from build123d import *

# Parameters (mm, degrees)
SKETCH1_W               = 147.6
SKETCH1_H               = 78.1
BOSS_EXTRUDE1_DEPTH     = 14.5
SKETCH2_W               = 112
SKETCH2_H               = 78.1
BOSS_EXTRUDE2_DEPTH     = 93.5
CUT_EXTRUDE1_REACH      = 200.87
CUT_EXTRUDE2_DEPTH      = 8.4
CUT_EXTRUDE2_DEPTH_BACK = 8.4
SKETCH4_R               = 6.5
CUT_EXTRUDE3_REACH      = 185.305
SKETCH5_R               = 4
SKETCH7_R               = 4
CUT_EXTRUDE4_DEPTH      = 199.870234166


with BuildPart() as part:
    # Sketch1 → Boss-Extrude1 (new body)
    with BuildSketch(Plane.XY):
        with Locations((73.8, 39.05)):
            Rectangle(SKETCH1_W, SKETCH1_H)
    extrude(amount=BOSS_EXTRUDE1_DEPTH)

    # Sketch2 → Boss-Extrude2 (add)
    with BuildSketch(Plane.XY.offset(14.5)):
        with Locations((73.8, 39.05)):
            Rectangle(SKETCH2_W, SKETCH2_H)
    extrude(amount=BOSS_EXTRUDE2_DEPTH)

    # Sketch3 → Cut-Extrude1 (cut, up to next)
    with BuildSketch(Plane(origin=(0, 78.1, 0), x_dir=(1, 0, 0), z_dir=(0, 1, 0)), mode=Mode.PRIVATE) as cut_extrude1_sk1:
        with BuildLine():
            Line((29.8, -84), (17.8, -84))
            Line((17.8, -84), (17.8, -108))
            Line((17.8, -108), (73.8, -108))
            ThreePointArc((73.8, -108), (48.740071828, -101.609868316), (29.8, -84))
        make_face()
    cut_extrude1_tool1 = extrude(cut_extrude1_sk1.sketch, amount=-CUT_EXTRUDE1_REACH, mode=Mode.PRIVATE) & part.part
    # Sketch3 → Cut-Extrude1 (cut, up to next)
    with BuildSketch(Plane(origin=(0, 78.1, 0), x_dir=(1, 0, 0), z_dir=(0, 1, 0)), mode=Mode.PRIVATE) as cut_extrude1_sk2:
        with BuildLine():
            Line((17.8, -53.866666667), (17.8, -57.466666667))
            Line((17.8, -57.466666667), (33.840520524, -57.466666667))
            ThreePointArc((33.840520524, -57.466666667), (113.8, -55.666666667), (33.840520524, -53.866666667))
            Line((33.840520524, -53.866666667), (17.8, -53.866666667))
        make_face()
    cut_extrude1_tool2 = extrude(cut_extrude1_sk2.sketch, amount=-CUT_EXTRUDE1_REACH, mode=Mode.PRIVATE) & part.part
    # Sketch3 → Cut-Extrude1 (cut, up to next)
    with BuildSketch(Plane(origin=(0, 78.1, 0), x_dir=(1, 0, 0), z_dir=(0, 1, 0)), mode=Mode.PRIVATE) as cut_extrude1_sk3:
        with BuildLine():
            ThreePointArc((117.8, -84), (98.859928172, -101.609868316), (73.8, -108))
            Line((73.8, -108), (129.8, -108))
            Line((129.8, -108), (129.8, -84))
            Line((129.8, -84), (117.8, -84))
        make_face()
    cut_extrude1_tool3 = extrude(cut_extrude1_sk3.sketch, amount=-CUT_EXTRUDE1_REACH, mode=Mode.PRIVATE) & part.part
    add(cut_extrude1_tool1.solids().sort_by_distance((32.341594, 78.1, 98.707997))[0], mode=Mode.SUBTRACT)
    add(cut_extrude1_tool2.solids().sort_by_distance((73.255815, 78.1, 55.666667))[0], mode=Mode.SUBTRACT)
    add(cut_extrude1_tool3.solids().sort_by_distance((115.258406, 78.1, 98.707997))[0], mode=Mode.SUBTRACT)

    # Sketch4 → Cut-Extrude2 (cut, two sides: drawn at the far end of the back side and taken through both)
    with BuildSketch(Plane.XY.offset(84).offset(-CUT_EXTRUDE2_DEPTH_BACK)):
        with Locations(Location((25.5, 61.05, 0), (0, 0, 311.417298986))):
            Circle(SKETCH4_R)
        with Locations(Location((25.5, 39.05, 0), (0, 0, 311.417298986))):
            Circle(SKETCH4_R)
        with Locations(Location((25.5, 17.05, 0), (0, 0, 180))):
            Circle(SKETCH4_R)
    extrude(amount=CUT_EXTRUDE2_DEPTH + CUT_EXTRUDE2_DEPTH_BACK, mode=Mode.SUBTRACT)

    # Sketch5 → Cut-Extrude3 (cut, up to next)
    with BuildSketch(Plane.XY.offset(75.6), mode=Mode.PRIVATE) as cut_extrude3_sk1:
        with Locations((25.5, 61.05)):
            Circle(SKETCH5_R)
    cut_extrude3_tool1 = extrude(cut_extrude3_sk1.sketch, amount=-CUT_EXTRUDE3_REACH, mode=Mode.PRIVATE) & part.part
    # Sketch5 → Cut-Extrude3 (cut, up to next)
    with BuildSketch(Plane.XY.offset(75.6), mode=Mode.PRIVATE) as cut_extrude3_sk2:
        with Locations((25.5, 39.05)):
            Circle(SKETCH5_R)
    cut_extrude3_tool2 = extrude(cut_extrude3_sk2.sketch, amount=-CUT_EXTRUDE3_REACH, mode=Mode.PRIVATE) & part.part
    # Sketch5 → Cut-Extrude3 (cut, up to next)
    with BuildSketch(Plane.XY.offset(75.6), mode=Mode.PRIVATE) as cut_extrude3_sk3:
        with Locations((25.5, 17.05)):
            Circle(SKETCH5_R)
    cut_extrude3_tool3 = extrude(cut_extrude3_sk3.sketch, amount=-CUT_EXTRUDE3_REACH, mode=Mode.PRIVATE) & part.part
    add(cut_extrude3_tool1.solids().sort_by_distance((25.5, 61.05, 75.6))[0], mode=Mode.SUBTRACT)
    add(cut_extrude3_tool2.solids().sort_by_distance((25.5, 39.05, 75.6))[0], mode=Mode.SUBTRACT)
    add(cut_extrude3_tool3.solids().sort_by_distance((25.5, 17.05, 75.6))[0], mode=Mode.SUBTRACT)

    # Sketch7 → Cut-Extrude4 (cut, through all)
    with BuildSketch(Plane(origin=(0, 0, 0), x_dir=(-1, 0, 0), z_dir=(0, 0, -1))):
        with Locations((-9, 63.1)):
            Circle(SKETCH7_R)
        with Locations((-9, 13.1)):
            Circle(SKETCH7_R)
        with Locations((-138.6, 13.1)):
            Circle(SKETCH7_R)
        with Locations((-138.6, 63.1)):
            Circle(SKETCH7_R)
    extrude(amount=-CUT_EXTRUDE4_DEPTH, mode=Mode.SUBTRACT)


solid = part.part
Source: CAD feature listing. Evaluate the final solid. Frame: model axes, mm. A direction names the side the tool comes from. Round coordinates to 2 decimals unless told otherwise and drop trailing zeros. Loops run counter-clockwise (first coordinate to the right, second up) from the corner with the lowest first, then second, coordinate; pieces in that order, holes last. Notation, with made-up numbers: (34.5, 0.5) - (56.5, 0.5) arc R18 cw to (56.5, 22.5) - close; hole circle Ø6 at (10.5, -14). An arc over 180 degrees is marked (long way). Write item = value, one per line. Start each with the question number.
Item 1: Reachability of faces 4 (the face through (31, 40, 57.467)), 5 (the face through (24.979, 43.016, 66.66)), 6 (the face through (17.8, 39, 34)) from +Z, -Z, +X, -X, +Y, -Y: full face, straight path, thin tool, end or side. Return the list, or none.
Item 2: Section query B-B on z = 31.5. Output: boundary loops of the cut face in (x, y).
Item 3: Section query A-A on x = 9. Output: boundary loops of the cut face in (y, z), plus the area to 3 significant figures.
Item 4: Section query D-D on y = 61.05. Count the separate pieces of the cut face and the enclosed holes in it, plus the area to 3 significant figures.
Item 5: Mould query, pull axis Z, two halves, no side actions, for faces 1 (the face through (26, 40, 53.867)), 2 (the face through (21, 17, 75.6)), 3 (the face through (0, 39, 7)). Classes: released by +Z, released by -Z, zero draft, split by the parting line, or undercut.
Item 6: Material intervals for line 1 (Y direction, x = 138.6, z = 3.75); line 2 (Y direction, x = 25, z = 78); line 3 (Z direction, x = 27.5, y = 72.5), sorted ascending.
Item 7: Section query C-C on y = 39.05. Output: boundary loops of the cut face in (x, z), plus the area to 3 significant figures.
Item 8: First-contact query: pin 1 Ø9 at (x, y) = (25.5, 17.05) entering from +Z; pin 2 Ø10 at (x, y) = (107, 51) entering from +Z; pin 3 Ø21 at (x, y) = (25.5, 17.05) entering from +Z. Flat tips, straight axial feed; report the tip coordinate or a pass-through.
Results list:
q1.face_4 = -X, +Y, -Y
q1.face_5 = +Z
q1.face_6 = +Z, -X, +Y, -Y
q2.outline = (17.8, 0) - (41.93, 0) - (41.93, 78.1) - (17.8, 78.1) - close; (105.67, 0) - (129.8, 0) - (129.8, 78.1) - (105.67, 78.1) - close
q3.outline = (0, 0) - (9.1, 0) - (9.1, 14.5) - (0, 14.5) - close; (17.1, 0) - (59.1, 0) - (59.1, 14.5) - (17.1, 14.5) - close; (67.1, 0) - (78.1, 0) - (78.1, 14.5) - (67.1, 14.5) - close
q3.area = 900 mm²
q4.separate_pieces = 4
q4.enclosed_holes = 0
q4.area = 5,870 mm²
q5.face_1 = undercut
q5.face_2 = released by +Z
q5.face_3 = zero draft
q6.line_1 = 0 to 9.1, 17.1 to 59.1, 67.1 to 78.1
q6.line_2 = 0 to 10.57, 23.53 to 32.57, 45.53 to 54.57, 67.53 to 78.1
q6.line_3 = 0 to 53.87, 57.47 to 84
q7.outline = (0, 0) - (147.6, 0) - (147.6, 14.5) - (129.8, 14.5) - (129.8, 84) - (117.8, 84) arc R52.33 ccw to (32, 87.16) - (32, 75.6) - (29.5, 75.6) - (29.5, 57.47) - (33.84, 57.47) arc R40 cw (long way) to (33.84, 53.87) - (17.8, 53.87) - (17.8, 14.5) - (0, 14.5) - close; (17.8, 57.47) - (21.5, 57.47) - (21.5, 75.6) - (19, 75.6) - (19, 84) - (17.8, 84) - close
q7.area = 6,070 mm²
q8.pin_1 = 75.6
q8.pin_2 = 99.75
q8.pin_3 = 91.86
